Design review of the part built by this model. Coordinates are the model's own, in mm. A direction names the side the tool comes from. Coordinates: 2 decimals unless noted, no trailing zeros. Loops run counter-clockwise (first coordinate to the right, second up) from the corner with the lowest first, then second, coordinate; pieces in that order, holes last. Notation, with made-up numbers: (-12, 20.25) - (22, 20.25) arc R14 cw to (22, 32.25) - close; hole circle Ø1 at (6.5, 56). An arc over 180 degrees is marked (long way). Answer in a Markdown table with one row per item. Add a question column.
(1) We need section B-B, the plane z = 38. Give the number of separate pieces and of enclosed holes in the cut face, plus the area to 3 significant figures.
(2) We need section A-A, the plane y = -35. Write out the cut boundary in (x, z).
(3) Clearance check with flat-ended pins moving along their axes: pin 1 (6 mm diameter, centred on x = -9.18, y = -18.33, fed in from -Z); pin 2 (3.5 mm diameter, centred on x = -11.28, y = 17.11, fed in from -Z). State where each tip first meets the part, or that it passes through.
(4) To check wall thickness, follow L1, parallel to X at y = 35, z = 42.25; L2, parallel to Y at x = 22.5, z = 37. State the ranges of each line that lie inside material, in increasing order. Write a range as [from, to].
(5) For faces 1 (the face through (-42, 1, 40)), 2 (the face through (17.966, 1.326, 37.782)), list the 3-axis set-ups (+Z, -Z, +X, -X, +Y, -Y) from which the entire face can be reached by the end or side of a thin tool; tool diameter is ignored.
(6) The part is to be moulded in two halves that separate along Y. For faces 3 (the face through (40.289, 40.196, 39.631)), 4 (the face through (-9.72, -20.77, 37.78)), 5 (the face through (42, -1, 40)), 6 (the face through (-40.289, -40.196, 39.631)), say which applies: released by +Y, released by -Y, zero draft, split by the parting line, or undercut.
from build123d import *

# Parameters (mm, degrees)
PLACA_SOPORTE_M1_START             = 36.5
PLACA_SOPORTE_M1_DEPTH             = 6.35
BARRENOS_SEPARADORES_Y_MOTOR_START = 36.5
CROQUIS2_R                         = 2.25
CROQUIS2_R_2                       = 1.45
CROQUIS2_R_3                       = 8
BARRENOS_SEPARADORES_Y_MOTOR_DEPTH = 6.35
REFRENTADO_M2_5_START              = 36.5
CROQUIS3_R                         = 2.5
REFRENTADO_M2_5_DEPTH              = 2.6


with BuildPart() as part:
    # Croquis1 → Placa_soporte_M1 (new body)
    with BuildSketch(Plane.XY.offset(PLACA_SOPORTE_M1_START)):
        with BuildLine():
            Line((-36, -42), (36, -42))
            ThreePointArc((36, -42), (40.242640687, -40.242640687), (42, -36))
            Line((42, -36), (42, 36))
            ThreePointArc((42, 36), (40.242640687, 40.242640687), (36, 42))
            Line((36, 42), (-36, 42))
            ThreePointArc((-36, 42), (-40.242640687, 40.242640687), (-42, 36))
            Line((-42, 36), (-42, -36))
            ThreePointArc((-42, -36), (-40.242640687, -40.242640687), (-36, -42))
        make_face()
    extrude(amount=PLACA_SOPORTE_M1_DEPTH)

    # Croquis2 → Barrenos_separadores_y_motor (cut)
    with BuildSketch(Plane.XY.offset(BARRENOS_SEPARADORES_Y_MOTOR_START)):
        with Locations((-36, -36)):
            Circle(CROQUIS2_R)
        with Locations((-36, 36)):
            Circle(CROQUIS2_R)
        with Locations((36, -36)):
            Circle(CROQUIS2_R)
        with Locations((36, 36)):
            Circle(CROQUIS2_R)
        with Locations((20.463916472, 1.215780658)):
            Circle(CROQUIS2_R_2)
        with Locations((9.179061301, 18.330161855)):
            Circle(CROQUIS2_R_2)
        with Locations((-11.284855172, 17.114381197)):
            Circle(CROQUIS2_R_2)
        with Locations((-20.463916472, -1.215780658)):
            Circle(CROQUIS2_R_2)
        with Locations((-9.179061301, -18.330161855)):
            Circle(CROQUIS2_R_2)
        with Locations((11.284855172, -17.114381197)):
            Circle(CROQUIS2_R_2)
        Circle(CROQUIS2_R_3)
    extrude(amount=BARRENOS_SEPARADORES_Y_MOTOR_DEPTH, mode=Mode.SUBTRACT)

    # Croquis3 → Refrentado_M2-5 (cut)
    with BuildSketch(Plane.XY.offset(REFRENTADO_M2_5_START)):
        with Locations((20.463916472, 1.215780658)):
            Circle(CROQUIS3_R)
        with Locations((9.179061301, 18.330161855)):
            Circle(CROQUIS3_R)
        with Locations((-11.284855172, 17.114381197)):
            Circle(CROQUIS3_R)
        with Locations((-20.463916472, -1.215780658)):
            Circle(CROQUIS3_R)
        with Locations((-9.179061301, -18.330161855)):
            Circle(CROQUIS3_R)
        with Locations((11.284855172, -17.114381197)):
            Circle(CROQUIS3_R)
    extrude(amount=REFRENTADO_M2_5_DEPTH, mode=Mode.SUBTRACT)


solid = part.part
Responses:
| question | item | result |
|---|---|---|
| 1 | separate pieces | 1 |
| 1 | enclosed holes | 11 |
| 1 | area | 6,640 mm2 |
| 2 | outline | (-42, 36.5) - (-38.02, 36.5) - (-38.02, 42.85) - (-42, 42.85) - close; (-33.98, 36.5) - (33.98, 36.5) - (33.98, 42.85) - (-33.98, 42.85) - close; (38.02, 36.5) - (42, 36.5) - (42, 42.85) - (38.02, 42.85) - close |
| 3 | pin 1 | stops at z = 36.5 |
| 3 | pin 2 | stops at z = 39.1 |
| 4 | L1 | x = [-42, -38.02], [-33.98, 33.98], [38.02, 42] |
| 4 | L2 | y = [-42, -0.23], [2.67, 42] |
| 5 | face 1 | +Z, -Z, -X, +Y, -Y |
| 5 | face 2 | -Z |
| 6 | face 3 | released by +Y |
| 6 | face 4 | undercut |
| 6 | face 5 | zero draft |
| 6 | face 6 | released by -Y |
